from build123d import *

# Parameters (mm, degrees)
PAD_DEPTH = 15
FILLET_R  = 1


with BuildPart() as part:
    # Sketch → Pad (new body)
    with BuildSketch(Plane.XY):
        with BuildLine():
            ThreePointArc((12.452434, 1.089447), (-12.5, 0), (12.452434, -1.089447))
            Line((12.452434, -1.089447), (17.931505, -1.568803))
            ThreePointArc((17.931505, 1.568803), (-18, 0), (17.931505, -1.568803))
            Line((12.452434, 1.089447), (17.931505, 1.568803))
        make_face()
    extrude(amount=PAD_DEPTH)

    # Fillet
    fillet_edges = [part.edges().sort_by_distance(p)[0] for p in [
        (12.452434, 1.089447, 7.5),
        (12.452434, -1.089447, 7.5),
    ]]
    fillet(fillet_edges, radius=FILLET_R)


solid = part.part
Verification items for the finished model (mm, model axes). A direction names the side the tool comes from. Coordinates: 2 decimals unless noted, no trailing zeros. Order: outer loops, then holes, each group sorted by start corner. A loop starts at its lowest first (then second) coordinate and runs counter-clockwise, first axis right, second up. Notation, with made-up numbers: M -30.75,50 L 9.25,50 A35 ccw 9.25,83 Z; hole C 36,26.25 d1. An arc over 180 degrees is marked long. Return JSON: item names as keys, results as strings.
1) Cross-section at A-A, the plane x = 0. Record the boundary of the cut face in (y, z).
Answer list:
{"outline": "M -18,0 L -12.5,0 L -12.5,15 L -18,15 Z; M 12.5,0 L 18,0 L 18,15 L 12.5,15 Z"}
2) Thickness scan on L1, parallel to Y at x = 0, z = 6.75; L2, parallel to Y at x = -4.5, z = 12.5; L3, parallel to X at y = 8, z = 9. Record the ranges inside material, lowest first. Write a range as [from, to].
Answer list:
{"L1": "[-18, -12.5], [12.5, 18]", "L2": "[-17.43, -11.66], [11.66, 17.43]", "L3": "[-16.12, -9.6], [9.6, 16.12]"}
3) Cross-section at D-D, the plane x = -10. Record the boundary of the cut face in (y, z).
Answer list:
{"outline": "M -14.97,0 L -7.5,0 L -7.5,15 L -14.97,15 Z; M 7.5,0 L 14.97,0 L 14.97,15 L 7.5,15 Z"}
4) Gauge pin test, flat ends, axial feed: pin 1 (4 mm diameter, centred on y = 12.5, z = 5.5, fed in from +X); pin 2 (3 mm diameter, centred on y = 5.5, z = 8, fed in from +X); pin 3 (1.5 mm diameter, centred on y = -4.5, z = 6, fed in from -X). Record the tip position at first contact, or that the pin passes through.
Answer list:
{"pin 1": "x = 14.62", "pin 2": "x = 17.55", "pin 3": "x = -17.61"}
5) Release check for a two-part mould opening along Y. For faces 4 (the flat face through (-3.8, 12.3, 15)), 5 (the cylindrical face through (-17.984, 0.769, 7.395)), 6 (the flat face through (15.64, -1.37, 7.4)) record: +Y half, -Y half, draft (parallel to the pull), parting line (faces both ways), or undercut.
Answer list:
{"face 4": "draft", "face 5": "parting line", "face 6": "undercut"}
6) Access from +Z, -Z, +X, -X, +Y, -Y to the whole of each face (thin tool, end or side, straight path). Record for faces 1 (the cylindrical face through (12.7, -1.39, 7.6)), 2 (the flat face through (15.64, 1.37, 7.4)), 3 (the flat face through (-3.8, 12.3, 0)).
Answer list:
{"face 1": "+Z, -Z", "face 2": "+Z, -Z, +X", "face 3": "-Z, +X, -X, +Y, -Y"}
7) Cross-section at C-C, the plane y = 0. Record the boundary of the cut face in (x, z).
Answer list:
{"outline": "M -18,0 L -12.5,0 L -12.5,15 L -18,15 Z"}
8) Cross-section at B-B, the plane z = 6.25. Record the boundary of the cut face in (x, y).
Answer list:
{"outline": "M 12.34,-2.01 A12.5 cw long 12.34,2.01 A1 ccw 13.41,1.17 L 17.93,1.57 A18 ccw long 17.93,-1.57 L 13.41,-1.17 A1 ccw Z"}
